```python
from build123d import *

# Parameters (mm, degrees)
BOSS_EXTRUDE2_DEPTH                            = 5.08
CUT_EXTRUDE1_DEPTH                             = 38.862
CSK_FOR_1_4_FLAT_HEAD_MACHINE_SCREW_2_COUNT    = 2
CSK_FOR_1_4_FLAT_HEAD_MACHINE_SCREW_2_PITCH    = 81.915
CSK_FOR_1_4_FLAT_HEAD_MACHINE_SCREW_3_AT_COUNT = 2
CSK_FOR_1_4_FLAT_HEAD_MACHINE_SCREW_3_AT_PITCH = 63.5


with BuildPart() as part:
    # Sketch1 → Boss-Extrude2 (new body)
    with BuildSketch(Plane.XY):
        with BuildLine():
            Line((-95.25, -48.631740263), (-234.95, -48.631740263))
            ThreePointArc((-234.95, -48.631740263), (-266.7, -16.881740263), (-234.95, 14.868259737))
            Line((-234.95, 14.868259737), (-95.25, 14.868259737))
            ThreePointArc((-95.25, 14.868259737), (-63.5, -16.881740263), (-95.25, -48.631740263))
        make_face()
    extrude(amount=BOSS_EXTRUDE2_DEPTH)

    # Sketch2 → Cut-Extrude1 (cut)
    with BuildSketch(Plane(origin=(0, 0, 0), x_dir=(-1, 0, 0), z_dir=(0, 0, -1))):
        with BuildLine():
            Line((227.965, -31.613740263), (102.235, -31.613740263))
            ThreePointArc((102.235, -31.613740263), (87.503, -16.881740263), (102.235, -2.149740263))
            Line((102.235, -2.149740263), (227.965, -2.149740263))
            ThreePointArc((227.965, -2.149740263), (242.697, -16.881740263), (227.965, -31.613740263))
        make_face()
    extrude(amount=-CUT_EXTRUDE1_DEPTH, mode=Mode.SUBTRACT)

    # Sketch8 → CSK for 1_4 Flat Head Machine Screw _100 (revolve, cut)
    with BuildSketch(Plane(origin=(-127.635, 6.359259737, 0), x_dir=(0, 1, 0), z_dir=(1, 0, 0))):
        Polygon((0, 0), (0, 5.08), (3.3782, 5.08), (3.3782, 2.568232241), (6.4389, 0), align=None)
    csk_for_1_4_flat_head_machine_screw_100 = revolve(axis=Axis((-127.635, 6.359259737, -6.35), (0, 0, 1)), mode=Mode.SUBTRACT)

    # CSK for 1_4 Flat Head Machine Screw  2: CSK for 1_4 Flat Head Machine Screw _100 ×2
    with Locations(*[(-i * CSK_FOR_1_4_FLAT_HEAD_MACHINE_SCREW_2_PITCH, 0, 0) for i in range(1, CSK_FOR_1_4_FLAT_HEAD_MACHINE_SCREW_2_COUNT)]):
        add(csk_for_1_4_flat_head_machine_screw_100, mode=Mode.SUBTRACT)

    # Sketch9 → CSK for 1_4 Flat Head Machine Screw  3 (revolve, cut)
    with BuildSketch(Plane(origin=(-111.76, -40.122740263, 0), x_dir=(0, 1, 0), z_dir=(1, 0, 0))):
        Polygon((0, 0), (0, 5.08), (3.3782, 5.08), (3.3782, 2.568232241), (6.4389, 0), align=None)
    csk_for_1_4_flat_head_machine_screw_3 = revolve(axis=Axis((-111.76, -40.122740263, -6.35), (0, 0, 1)), mode=Mode.SUBTRACT)

    # CSK for 1_4 Flat Head Machine Screw 3 at: CSK for 1_4 Flat Head Machine Screw  3 ×2
    with Locations(*[(-i * CSK_FOR_1_4_FLAT_HEAD_MACHINE_SCREW_3_AT_PITCH, 0, 0) for i in range(1, CSK_FOR_1_4_FLAT_HEAD_MACHINE_SCREW_3_AT_COUNT)]):
        add(csk_for_1_4_flat_head_machine_screw_3, mode=Mode.SUBTRACT)

    # Sketch10 → CSK for 1_4 Flat Head Machine Screw  4 (revolve, cut)
    with BuildSketch(Plane(origin=(-238.76, -40.122740263, 0), x_dir=(0, 1, 0), z_dir=(1, 0, 0))):
        Polygon((0, 0), (0, 5.08), (3.3782, 5.08), (3.3782, 2.568232241), (6.4389, 0), align=None)
    revolve(axis=Axis((-238.76, -40.122740263, -6.35), (0, 0, 1)), mode=Mode.SUBTRACT)


solid = part.part
```
Can you work these out from the model? Positions are in its coordinate system, mm. A direction names the side the tool comes from. Coordinates: 2 decimals unless noted, no trailing zeros. Loops run counter-clockwise (first coordinate to the right, second up) from the corner with the lowest first, then second, coordinate; pieces in that order, holes last.
1) Imagine slicing it at A-A on x = -209.55. List the corners of the cut face in (y, z) for me, plus the area to 3 significant figures.
2) Imagine slicing it at D-D on x = -238.76. List the corners of the cut face in (y, z) for me.
3) For pin 1 (2 mm diameter, centred on x = -243.5, z = 3, fed in from -Y); pin 2 (2 mm diameter, centred on y = 3, z = 3, fed in from +X); pin 3 (1.5 mm diameter, centred on y = -30.5, z = 2.5, fed in from +X); pin 4 (6 mm diameter, centred on x = -103, y = -26.5, fed in from +Z), each with a flat end and sliding along its axis, tell me the tip position at first contact or that it passes through.
4) Which directions (+Z, -Z, +X, -X, +Y, -Y) give clear straight access to the entire face, cutting with the end or side of a thin tool? Please do faces 5 (the flat face through (-166, -31.614, 3)), 6 (the conical face through (-131.17, 5.89, 2.41)).
5) Imagine slicing it at B-B on x = -93.5. List the corners of the cut face in (y, z) for me, plus the area to 3 significant figures.
6) I need wall thicknesses on probe 1 along Y at (x, z) = (-209.55, 4.3); probe 2 along Y at (x, z) = (-187, 0.6); probe 3 along Y at (x, z) = (-175.26, 4.2). Which ranges of each line are inside material? Lowest first, please.
7) Imagine slicing it at C-C on y = -16. List the corners of the cut face in (x, z) for me.
8) Thinking about a two-plate mould opening in Y: for faces 1 (the cylindrical face through (-87.507, -17.206, 2.504)), 2 (the flat face through (-166, 14.868, 3)), 3 (the cylindrical face through (-63.508, -16.184, 2.504)), 4 (the flat face through (-164, -2.15, 3)), which applies, pulls with the +Y half, pulls with the -Y half, needs draft (parallel to the pull), parting line crosses it, or undercut?
Completed:
1. outline: (-48.63, 0) - (-31.61, 0) - (-31.61, 5.08) - (-48.63, 5.08) - close; (-2.15, 0) - (-0.08, 0) - (2.98, 2.57) - (2.98, 5.08) - (-2.15, 5.08) - close; (9.74, 2.57) - (12.8, 0) - (14.87, 0) - (14.87, 5.08) - (9.74, 5.08) - close
1. area: 131 mm2
2. outline: (-48.4, 0) - (-46.56, 0) - (-43.5, 2.57) - (-43.5, 5.08) - (-48.4, 5.08) - close; (-36.74, 2.57) - (-33.68, 0) - (-26.91, 0) - (-26.91, 5.08) - (-36.74, 5.08) - close; (-6.86, 0) - (14.64, 0) - (14.64, 5.08) - (-6.86, 5.08) - close
3. pin 1: stops at y = -47.72
3. pin 2: stops at x = -69.72
3. pin 3: stops at x = -66.22
3. pin 4: passes through
4. face 5: +Z, -Z
4. face 6: -Z
5. outline: (-48.58, 0) - (-28.74, 0) - (-28.74, 5.08) - (-48.58, 5.08) - close; (-5.02, 0) - (14.82, 0) - (14.82, 5.08) - (-5.02, 5.08) - close
5. area: 202 mm2
6. probe 1: y = -48.63 to -31.61, -2.15 to 2.98, 9.74 to 14.87
6. probe 2: y = -48.63 to -31.61, -2.15 to 14.87
6. probe 3: y = -48.63 to -43.5, -36.74 to -31.61, -2.15 to 14.87
7. outline: (-266.69, 0) - (-242.67, 0) - (-242.67, 5.08) - (-266.69, 5.08) - close; (-87.53, 0) - (-63.51, 0) - (-63.51, 5.08) - (-87.53, 5.08) - close
8. face 1: undercut
8. face 2: pulls with the +Y half
8. face 3: parting line crosses it
8. face 4: undercut
